Design review of the part shown in the three views and the two pictorial views. Dimensions are in mm from the part's minimum x, y and z. A direction names the side the tool comes from. Give positions to 0.01 mm unless a question says otherwise; leave off trailing zeros. Loops run counter-clockwise (first coordinate to the right, second up) from the corner with the lowest first, then second, coordinate; pieces in that order, holes last.
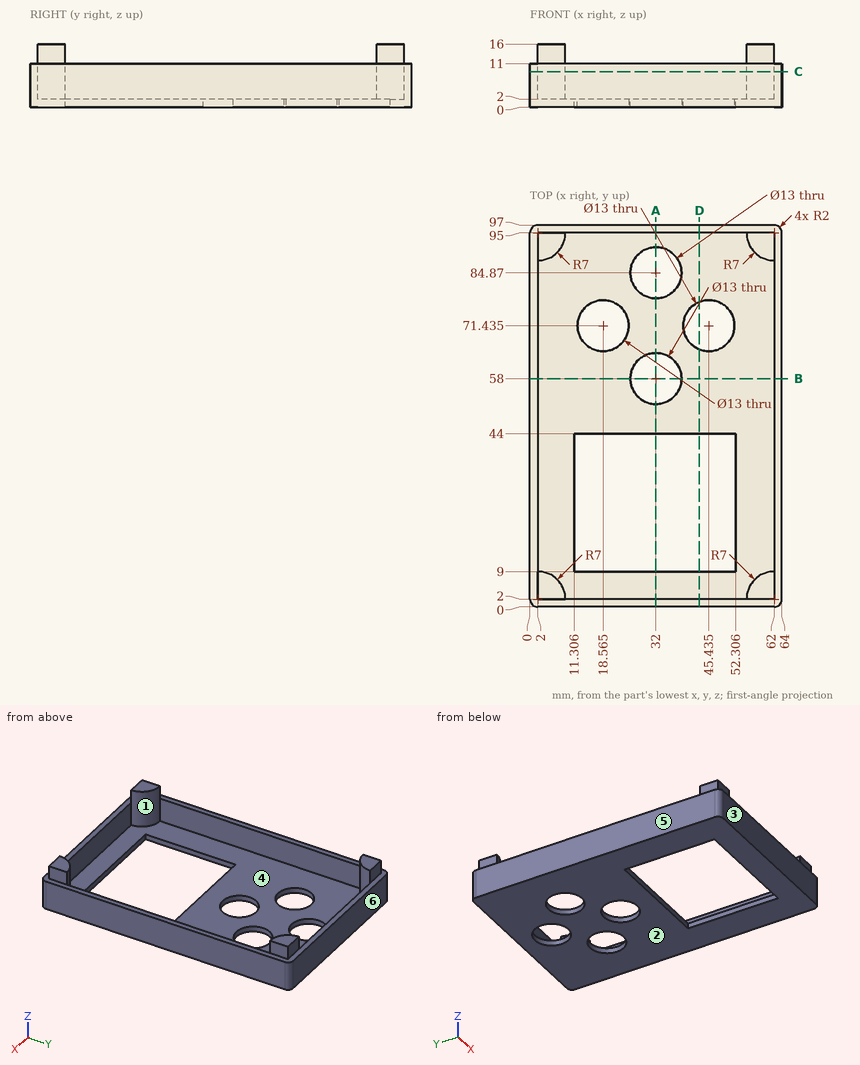
Q1. Consider section D-D on x = 43. Give the boundary of the cut face in (y, z).
Answers:
outline: (0, 0) - (9, 0) - (9, 2) - (2, 2) - (2, 11) - (0, 11) - close; (44, 0) - (65.41, 0) - (65.41, 2) - (44, 2) - close; (77.46, 0) - (97, 0) - (97, 11) - (95, 11) - (95, 2) - (77.46, 2) - close
Q2. Machinability: for the marked faces 1 and 2, which of the approach directions +Z, -Z, +X, -X, +Y, -Y give a long, thin tool a straight path to every point of the face, cutting with its end or side? Answer none if there is none.
Answers:
face 1: +Z
face 2: -Z, +X, -X, +Y, -Y
Q3. For probe 1 along Y at (x, z) = (32, 0.4); probe 2 along Y at (x, z) = (16.5, 7); probe 3 along X at (y, z) = (11, 7.25), list the stretches that pass through material, from the lowest coordinate up.
Answers:
probe 1: y = 0 to 9, 44 to 51.5, 64.5 to 78.37, 91.37 to 97
probe 2: y = 0 to 2, 95 to 97
probe 3: x = 0 to 2, 62 to 64
Q4. Consider section A-A on x = 32. Give the boundary of the cut face in (y, z).
Answers:
outline: (0, 0) - (9, 0) - (9, 2) - (2, 2) - (2, 11) - (0, 11) - close; (44, 0) - (51.5, 0) - (51.5, 2) - (44, 2) - close; (64.5, 0) - (78.37, 0) - (78.37, 2) - (64.5, 2) - close; (91.37, 0) - (97, 0) - (97, 11) - (95, 11) - (95, 2) - (91.37, 2) - close
Q5. Consider section C-C on z = 9. Give the boundary of the cut face in (x, y).
Answers:
outline: (0, 2) arc R2 ccw to (2, 0) - (62, 0) arc R2 ccw to (64, 2) - (64, 95) arc R2 ccw to (62, 97) - (2, 97) arc R2 ccw to (0, 95) - close; hole (2, 9) arc R7 cw to (9, 2) - (55, 2) arc R7 cw to (62, 9) - (62, 88) arc R7 cw to (55, 95) - (9, 95) arc R7 cw to (2, 88) - close
Q6. Consider section B-B on y = 58. Give the boundary of the cut face in (x, z).
Answers:
outline: (0, 0) - (25.5, 0) - (25.5, 2) - (2, 2) - (2, 11) - (0, 11) - close; (38.5, 0) - (64, 0) - (64, 11) - (62, 11) - (62, 2) - (38.5, 2) - close
Q7. Mouldability with a two-part tool opening along Y and no side actions: class the marked faces 3, 4, 5 and 6 as +Y half, -Y half, draft (parallel to the pull), parting line (faces both ways), or undercut.
Answers:
face 3: -Y half
face 4: undercut
face 5: draft
face 6: +Y half
Q8. For pin 1 Ø1.5 at (y, z) = (4, 13.5) entering from +X; pin 2 Ø12 at (x, y) = (37.5, 44.5) entering from +Z; pin 3 Ø5.5 at (y, z) = (6.5, 14.5) entering from -X, all flat-tipped, find the tip position at first contact; note any pin that passes through.
Answers:
pin 1: stops at x = 62
pin 2: stops at z = 2
pin 3: stops at x = 2
